from build123d import *

# Parameters (mm, degrees)
ESTRUSIONE_ESTRUSIONE1_DEPTH = 1000


with BuildPart() as part:
    # Schizzo1 → Estrusione-Estrusione1 (new body)
    with BuildSketch(Plane(origin=(0, 0, 0), x_dir=(0, -1, 0), z_dir=(-1, 0, 0))):
        with BuildLine():
            Line((-10.05312229, 8.25), (-6, 4.19687771))
            Line((-6, 4.19687771), (-6, 0.91961524))
            Line((-6, 0.91961524), (-5.469059893, -2e-09))
            Line((-5.469059893, -2e-09), (-6, -0.91961524))
            Line((-6, -0.91961524), (-6, -4.19687771))
            Line((-6, -4.19687771), (-10.05312229, -8.25))
            Line((-10.05312229, -8.25), (-12.80312305, -8.25))
            Line((-12.80312305, -8.25), (-12.8, -4))
            Line((-12.8, -4), (-14.5, -4))
            Line((-14.5, -4), (-14.5, -4.5))
            Line((-14.5, -4.5), (-15, -4.5))
            Line((-15, -4.5), (-15, -13))
            ThreePointArc((-15, -13), (-14.414213562, -14.414213562), (-13, -15))
            Line((-13, -15), (-4.5, -15))
            Line((-4.5, -15), (-4.5, -14.5))
            Line((-4.5, -14.5), (-4, -14.5))
            Line((-4, -14.5), (-4, -12.8))
            Line((-4, -12.8), (-8.25, -12.80312305))
            Line((-8.25, -12.80312305), (-8.25, -10.05312229))
            Line((-8.25, -10.05312229), (-4.19687771, -6))
            Line((-4.19687771, -6), (-0.91961524, -6))
            Line((-0.91961524, -6), (2e-09, -5.469059893))
            Line((2e-09, -5.469059893), (0.91961524, -6))
            Line((0.91961524, -6), (4.19687771, -6))
            Line((4.19687771, -6), (8.25, -10.05312229))
            Line((8.25, -10.05312229), (8.25, -12.80312305))
            Line((8.25, -12.80312305), (4, -12.8))
            Line((4, -12.8), (4, -14.5))
            Line((4, -14.5), (4.5, -14.5))
            Line((4.5, -14.5), (4.5, -15))
            Line((4.5, -15), (13, -15))
            ThreePointArc((13, -15), (14.414213562, -14.414213562), (15, -13))
            Line((15, -13), (15, -4.5))
            Line((15, -4.5), (14.5, -4.5))
            Line((14.5, -4.5), (14.5, -4))
            Line((14.5, -4), (12.8, -4))
            Line((12.8, -4), (12.80312305, -8.25))
            Line((12.80312305, -8.25), (10.05312229, -8.25))
            Line((10.05312229, -8.25), (6, -4.19687771))
            Line((6, -4.19687771), (6, -0.91961524))
            Line((6, -0.91961524), (5.469059893, -2e-09))
            Line((5.469059893, -2e-09), (6, 0.91961524))
            Line((6, 0.91961524), (6, 4.19687771))
            Line((6, 4.19687771), (10.05312229, 8.25))
            Line((10.05312229, 8.25), (12.80312305, 8.25))
            Line((12.80312305, 8.25), (12.8, 4))
            Line((12.8, 4), (14.5, 4))
            Line((14.5, 4), (14.5, 4.5))
            Line((14.5, 4.5), (15, 4.5))
            Line((15, 4.5), (15, 13))
            ThreePointArc((15, 13), (14.414213562, 14.414213562), (13, 15))
            Line((13, 15), (4.5, 15))
            Line((4.5, 15), (4.5, 14.5))
            Line((4.5, 14.5), (4, 14.5))
            Line((4, 14.5), (4, 12.8))
            Line((4, 12.8), (8.25, 12.80312305))
            Line((8.25, 12.80312305), (8.25, 10.05312229))
            Line((8.25, 10.05312229), (4.19687771, 6))
            Line((4.19687771, 6), (0.91961524, 6))
            Line((0.91961524, 6), (2e-09, 5.469059893))
            Line((2e-09, 5.469059893), (-0.91961524, 6))
            Line((-0.91961524, 6), (-4.19687771, 6))
            Line((-4.19687771, 6), (-8.25, 10.05312229))
            Line((-8.25, 10.05312229), (-8.25, 12.80312305))
            Line((-8.25, 12.80312305), (-4, 12.8))
            Line((-4, 12.8), (-4, 14.5))
            Line((-4, 14.5), (-4.5, 14.5))
            Line((-4.5, 14.5), (-4.5, 15))
            Line((-4.5, 15), (-13, 15))
            ThreePointArc((-13, 15), (-14.414213562, 14.414213562), (-15, 13))
            Line((-15, 13), (-15, 4.5))
            Line((-15, 4.5), (-14.5, 4.5))
            Line((-14.5, 4.5), (-14.5, 4))
            Line((-14.5, 4), (-12.8, 4))
            Line((-12.8, 4), (-12.80312305, 8.25))
            Line((-12.80312305, 8.25), (-10.05312229, 8.25))
        make_face()
        with BuildLine():
            Line((-3.117157854, 4.531371416), (-1.616767222, 3.272394195))
            ThreePointArc((-1.616767222, 3.272394195), (5e-09, 3.650000002), (1.616767231, 3.272394191))
            Line((1.616767231, 3.272394191), (3.117157862, 4.531371411))
            ThreePointArc((3.117157862, 4.531371411), (3.889087302, 3.889087292), (4.53137142, 3.11715785))
            Line((4.53137142, 3.11715785), (3.272394197, 1.616767219))
            ThreePointArc((3.272394197, 1.616767219), (3.650000003, -4e-09), (3.272394193, -1.616767225))
            Line((3.272394193, -1.616767225), (4.531371415, -3.117157856))
            ThreePointArc((4.531371415, -3.117157856), (3.889087297, -3.889087296), (3.117157857, -4.531371414))
            Line((3.117157857, -4.531371414), (1.616767227, -3.272394192))
            ThreePointArc((1.616767227, -3.272394192), (5e-09, -3.650000002), (-1.616767217, -3.272394197))
            Line((-1.616767217, -3.272394197), (-3.117157849, -4.531371419))
            ThreePointArc((-3.117157849, -4.531371419), (-3.889087291, -3.889087301), (-4.531371411, -3.117157861))
            Line((-4.531371411, -3.117157861), (-3.27239419, -1.61676723))
            ThreePointArc((-3.27239419, -1.61676723), (-3.650000002, -5e-09), (-3.272394194, 1.616767222))
            Line((-3.272394194, 1.616767222), (-4.531371416, 3.117157855))
            ThreePointArc((-4.531371416, 3.117157855), (-3.889087296, 3.889087297), (-3.117157854, 4.531371416))
        make_face(mode=Mode.SUBTRACT)
        with BuildLine():
            Line((12.85, 9.7), (10.7, 9.7))
            ThreePointArc((10.7, 9.7), (9.992893219, 9.992893219), (9.7, 10.7))
            Line((9.7, 10.7), (9.7, 12.85))
            ThreePointArc((9.7, 12.85), (9.992893219, 13.557106781), (10.7, 13.85))
            Line((10.7, 13.85), (12.85, 13.85))
            ThreePointArc((12.85, 13.85), (13.557106781, 13.557106781), (13.85, 12.85))
            Line((13.85, 12.85), (13.85, 10.7))
            ThreePointArc((13.85, 10.7), (13.557106781, 9.992893219), (12.85, 9.7))
        make_face(mode=Mode.SUBTRACT)
        with BuildLine():
            Line((-9.7, 12.85), (-9.7, 10.7))
            ThreePointArc((-9.7, 10.7), (-9.992893219, 9.992893219), (-10.7, 9.7))
            Line((-10.7, 9.7), (-12.85, 9.7))
            ThreePointArc((-12.85, 9.7), (-13.557106781, 9.992893219), (-13.85, 10.7))
            Line((-13.85, 10.7), (-13.85, 12.85))
            ThreePointArc((-13.85, 12.85), (-13.557106781, 13.557106781), (-12.85, 13.85))
            Line((-12.85, 13.85), (-10.7, 13.85))
            ThreePointArc((-10.7, 13.85), (-9.992893219, 13.557106781), (-9.7, 12.85))
        make_face(mode=Mode.SUBTRACT)
        with BuildLine():
            Line((-12.85, -9.7), (-10.7, -9.7))
            ThreePointArc((-10.7, -9.7), (-9.992893219, -9.992893219), (-9.7, -10.7))
            Line((-9.7, -10.7), (-9.7, -12.85))
            ThreePointArc((-9.7, -12.85), (-9.992893219, -13.557106781), (-10.7, -13.85))
            Line((-10.7, -13.85), (-12.85, -13.85))
            ThreePointArc((-12.85, -13.85), (-13.557106781, -13.557106781), (-13.85, -12.85))
            Line((-13.85, -12.85), (-13.85, -10.7))
            ThreePointArc((-13.85, -10.7), (-13.557106781, -9.992893219), (-12.85, -9.7))
        make_face(mode=Mode.SUBTRACT)
        with BuildLine():
            Line((9.7, -12.85), (9.7, -10.7))
            ThreePointArc((9.7, -10.7), (9.992893219, -9.992893219), (10.7, -9.7))
            Line((10.7, -9.7), (12.85, -9.7))
            ThreePointArc((12.85, -9.7), (13.557106781, -9.992893219), (13.85, -10.7))
            Line((13.85, -10.7), (13.85, -12.85))
            ThreePointArc((13.85, -12.85), (13.557106781, -13.557106781), (12.85, -13.85))
            Line((12.85, -13.85), (10.7, -13.85))
            ThreePointArc((10.7, -13.85), (9.992893219, -13.557106781), (9.7, -12.85))
        make_face(mode=Mode.SUBTRACT)
    extrude(amount=-ESTRUSIONE_ESTRUSIONE1_DEPTH)


solid = part.part
Input: part model. Units: mm. Frame: model coordinates. Coordinates: 2 decimals unless noted, no trailing zeros. Answer in a Markdown table with one row per item. Add a question column.
Item 1: Contact query for flat-ended pins moving along their axis: P1, Ø2, axis at x = 163.5, y = -2, coming from the -Z side; P2, Ø2, axis at y = 0.5, z = -3, coming from the +X side; P3, Ø0.8, axis at x = 682.5, y = -14, coming from the -Z side; P4, Ø1, axis at x = 399, z = 1, coming from the -Y side. Output: stop coordinate, or through.
Item 2: Line query: line 1 along Y through (x, z) = (814.5, 6.5); line 2 along Z through (x, y) = (147, 13); line 3 along Z through (x, y) = (584, -12.75). Output: solid intervals per line, ascending. Write a range as [from, to].
Item 3: Section query A-A on x = 364. State how many separate pieces and enclosed holes the cut face has, then the cut area to 3 significant figures.
Recorded:
| question | item | result |
|---|---|---|
| 1 | P1 | z = -6 |
| 1 | P2 | x = 1000 |
| 1 | P3 | z = -14.91 |
| 1 | P4 | y = -6 |
| 2 | line 1 | [-15, -12.8], [-8.3, -4.7], [4.7, 8.3], [12.8, 15] |
| 2 | line 2 | [-15, -13.84], [-9.71, -4], [4, 9.71], [13.84, 15] |
| 2 | line 3 | [-15, -13.85], [-9.7, -8.25], [8.25, 9.7], [13.85, 15] |
| 3 | separate pieces | 1 |
| 3 | enclosed holes | 5 |
| 3 | area | 316 mm^2 |
